Design review of the part shown in the three views and the two pictorial views. Dimensions are in mm from the part's minimum x, y and z. Round coordinates to 2 decimals unless told otherwise and drop trailing zeros. Order: outer loops, then holes, each group sorted by start corner. A loop starts at its lowest first (then second) coordinate and runs counter-clockwise, first axis right, second up.
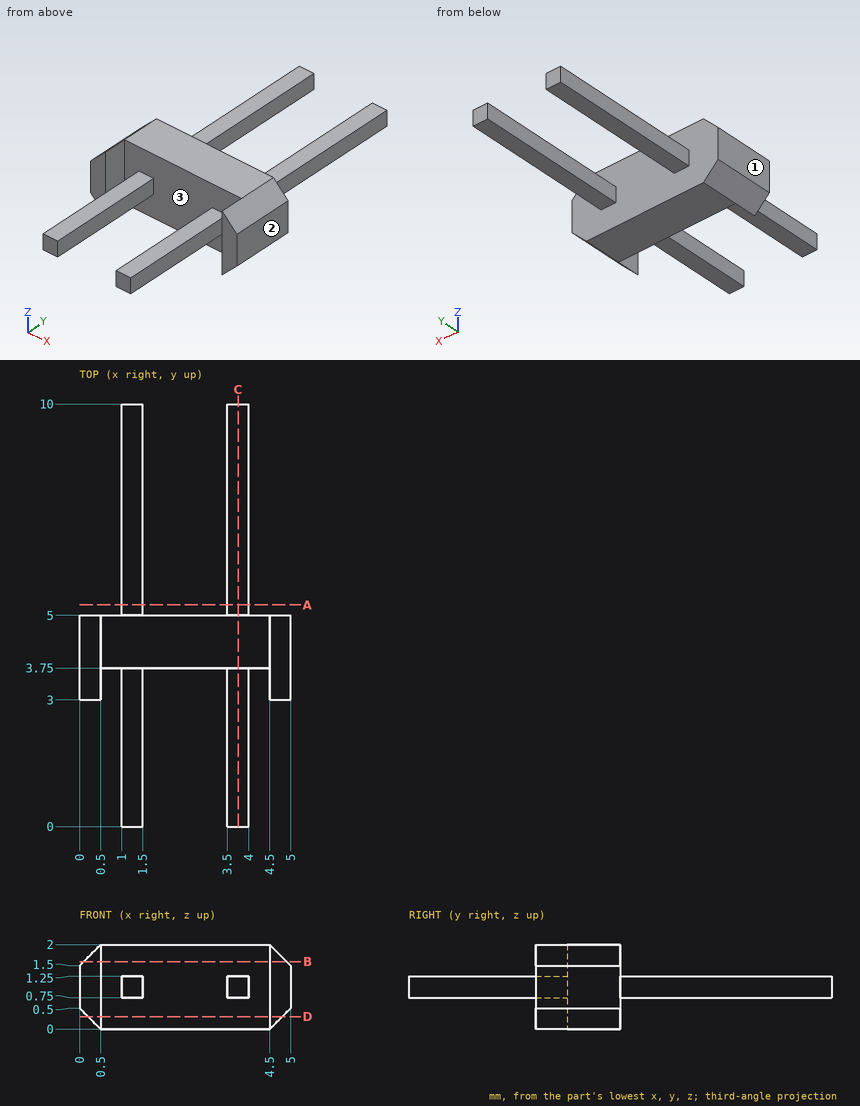
(1) Add section B-B on z = 1.6. Give the boundary of the cut face in (x, y).
(2) Wall thickness on L1, parallel to X at y = 5.5, z = 1.05; L2, parallel to Y at x = 2.55, z = 1.7; L3, parallel to Z at x = 3.9, y = 8.5: over which ranges is each line inside the solid? List them lowest first.
(3) Add section A-A on y = 5.25. Give the boundary of the cut face in (x, z).
(4) Add section C-C on x = 3.75. Give the boundary of the cut face in (y, z).
(5) Add section D-D on z = 0.3. Give the boundary of the cut face in (x, y).
(6) Clearance check with flat-ended pins moving along their axes: P1, Ø2, axis at x = 3, y = 8, coming from the -Z side; P2, Ø0.6, axis at y = 1, z = 1, coming from the -X side. State where each tip first meets the part, or that it passes through.
(7) Draft analysis for pull direction X (two halves, no side actions). For the marked faces 1, 2 and 3, state which applies: pulls with the +X half, pulls with the -X half, needs draft (parallel to the pull), parting line crosses it, or undercut.
Here are the results:
1. outline: (0.1, 3) - (0.5, 3) - (0.5, 3.75) - (4.5, 3.75) - (4.5, 3) - (4.9, 3) - (4.9, 5) - (0.1, 5) - close
2. L1: x = 1 to 1.5, 3.5 to 4
2. L2: y = 3.75 to 5
2. L3: z = 0.75 to 1.25
3. outline: (1, 0.75) - (1.5, 0.75) - (1.5, 1.25) - (1, 1.25) - close; (3.5, 0.75) - (4, 0.75) - (4, 1.25) - (3.5, 1.25) - close
4. outline: (0, 0.75) - (3.75, 0.75) - (3.75, 0) - (5, 0) - (5, 0.75) - (10, 0.75) - (10, 1.25) - (5, 1.25) - (5, 2) - (3.75, 2) - (3.75, 1.25) - (0, 1.25) - close
5. outline: (0.2, 3) - (0.5, 3) - (0.5, 3.75) - (4.5, 3.75) - (4.5, 3) - (4.8, 3) - (4.8, 5) - (0.2, 5) - close
6. P1: stops at z = 0.75
6. P2: stops at x = 1
7. face 1: pulls with the -X half
7. face 2: pulls with the +X half
7. face 3: undercut
